Here's how the part is built. I have some questions about the finished solid (model axes, mm). Face numbers are marked on the shaded views. A direction names the side the tool comes from. Coordinates: 2 decimals unless noted, no trailing zeros. Loops run counter-clockwise (first coordinate to the right, second up) from the corner with the lowest first, then second, coordinate; pieces in that order, holes last. Notation, with made-up numbers: M 18.5,-5.75 L 72.5,-5.75 A32 ccw 72.5,29.25 Z; hole C 77.5,-30 d2. An arc over 180 degrees is marked long. Use one line per item in the form item = value. Start each with the question number.
(1) Imagine slicing it at B-B, the plane x = -62. Please give me the cut outline in (y, z).
(2) On a 3-axis mill with a long thin cutter (end or side, diameter ignored), from which of +Z, -Z, +X, -X, +Y, -Y can I reach the whole of each face in a straight line? I mean the marked faces 5 and 6. Say none if no direction works.
(3) Imagine slicing it at D-D, the plane x = -77. Please give me the cut outline in (y, z).
(4) Please list where these lines run through material, in increasing order: L1, parallel to Z at x = -86, y = 3.9; L2, parallel to Z at x = -62, y = 1.55; L3, parallel to X at y = 2.85, z = -12.5.
(5) Imagine slicing it at A-A, the plane z = -12.5. Please give me the cut outline in (x, y), and give its area (3 significant figures).
(6) Imagine slicing it at C-C, the plane y = 3.8. State how many separate pieces and enclosed holes the cut face has, and give its area (3 significant figures).
(7) Thinking about a two-plate mould opening in X: for the marked faces 1, 2, 3 and 4, which applies, +X half, -X half, draft (parallel to the pull), parting line (faces both ways), or undercut?
(8) Will this pin go through, and if not, where does the flat tip stop? P1, Ø3, axis at y = 3, z = -64.5, coming from the +X side.
Autodesk Inventor part; units mm, degrees
ref_plane "YZ Plane" through (0, 0, 0) normal (1, 0, 0) x (0, 1, 0)
ref_plane "XZ Plane" through (0, 0, 0) normal (0, 1, 0) x (-1, 0, 0)
ref_plane "XY Plane" through (0, 0, 0) normal (0, 0, 1) x (1, 0, 0)
sketch "Sketch1" plane through (0, 0, 0) normal (0, 1, 0) x (-1, 0, 0)
  line L0 (0, 0) -> (105, 0)
  line L1 (105, 0) -> (105, -50)
  line L2 (105, -50) -> (0, -50)
  line L3 (0, -50) -> (0, 0)
  line L4 (0, 0) -> (0, -16.6667)
  line L5 (0, -16.6667) -> (11, -16.6667)
  dimension "d0" = 105
  dimension "d1" = 50
  dimension "d2" = 16.6667
  dimension "d3" = 11
extrude "Extrusion1" add sketch "Sketch1" along normal blind 6
sketch "Sketch3" plane through (0, 6, 0) normal (0, 1, 0) x (1, 0, 0)
  circle A0 centre (-20, 12.5) radius 2.75
  line L0 (0, 0) -> (0, 50)
  line L1 (-105, 0) -> (0, 0)
  circle A1 centre (-20, 37.5) radius 2.75
  dimension "d21" = 5.5
  dimension "d22" = 20
  dimension "d23" = 12.5
  dimension "d26" = 25
extrude "Extrusion3" cut sketch "Sketch3" against normal through all
sketch "Sketch4" plane through (0, 6, 0) normal (0, 1, 0) x (1, 0, 0)
  circle A0 centre (-20, 12.5) radius 2.75
  line L0 (-20, 12.5) -> (-78, 12.5)
  line L1 (-78, 12.5) -> (-88, 12.5) construction
  line L2 (-78, 15.25) -> (-88, 15.25)
  line L3 (-88, 9.75) -> (-78, 9.75)
  arc A1 (-78, 9.75) -> (-78, 15.25) centre (-78, 12.5) ccw
  arc A2 (-88, 15.25) -> (-88, 9.75) centre (-88, 12.5) ccw
  point P0 (0, 0)
  point P1 (-83, 12.5)
  dimension "d33" = 58
  dimension "d34" = 10
  dimension "d35" = 5.5
extrude "Extrusion4" cut sketch "Sketch4" against normal through all contours A1 L3 A2 L2
pattern_linear "Rectangular Pattern2" count 2 spacing 25 along (0, 0, -1) of "Extrusion4"
sketch "Sketch5" plane through (0, 0, -50) normal (0, 0, -1) x (-1, 0, 0)
  line L0 (105, 0) -> (105, 6)
  line L1 (105, 0) -> (0, 0)
  line L2 (105, 6) -> (75, 6)
  line L3 (75, 6) -> (75, 0)
  line L4 (75, 0) -> (105, 0)
  line L5 (105, 0) -> (105, 6)
  dimension "d45" = 30
extrude "Extrusion5" add sketch "Sketch5" along normal blind 25
sketch "Sketch6" plane through (0, 6, 0) normal (0, 1, 0) x (1, 0, 0)
  line L0 (-83, 60.5) -> (-83, 70.5) construction
  line L1 (-80.25, 60.5) -> (-80.25, 70.5)
  line L2 (-85.75, 70.5) -> (-85.75, 60.5)
  arc A0 (-85.75, 60.5) -> (-80.25, 60.5) centre (-83, 60.5) ccw
  arc A1 (-80.25, 70.5) -> (-85.75, 70.5) centre (-83, 70.5) ccw
  line L3 (-75, 50) -> (-75, 75)
  arc A2 (-88, 40.25) -> (-88, 34.75) centre (-88, 37.5) ccw
  point P0 (0, 0)
  point P1 (-83, 65.5)
  dimension "d48" = 10
  dimension "d49" = 5.5
  dimension "d50" = 8
  dimension "d51" = 28
extrude "Extrusion6" cut sketch "Sketch6" against normal through all
fillet "Fillet2" radius 5 6 edges at (-105, 3, 0) (0, 3, 0) (-75, 3, -75) (-105, 3, -75) (0, 3, -50) (-75, 3, -50)
sketch "Sketch7" plane through (0, 6, 0) normal (0, 1, 0) x (1, 0, 0)
  circle A0 centre (-20, 12.5) radius 2.75
  line L0 (-20, 12.5) -> (-42, 12.5)
  line L1 (-42, 12.5) -> (-62, 12.5)
  circle A1 centre (-62, 12.5) radius 2.75
  circle A2 centre (-42, 12.5) radius 2.75
  line L2 (0, 5) -> (0, 45)
  line L3 (0, 0) -> (0, 45)
  circle A3 centre (-42, 37.5) radius 2.75
  circle A4 centre (-62, 37.5) radius 2.75
  dimension "d55" = 22
  dimension "d56" = 20
  dimension "d57" = 5.5
  dimension "d58" = 5.5
  dimension "d61" = 25
extrude "Extrusion7" cut sketch "Sketch7" against normal through all contours A2 L1 L0 | L0 L1 A2 | A1 | A3 | A4
sketch "Sketch9" plane through (0, 6, 0) normal (0, 1, 0) x (1, 0, 0)
  point P0 (0, 0)
sketch "Sketch10" plane through (0, 6, 0) normal (0, 1, 0) x (1, 0, 0)
  circle A0 centre (-100, 70) radius 2.75
  line L0 (-100, 75) -> (-80, 75)
  line L1 (-105, 5) -> (-105, 70)
  circle A1 centre (-100, 5) radius 2.75
  line L2 (-100, 0) -> (-5, 0)
  circle A2 centre (-5, 45) radius 2.75
  line L3 (-5, 50) -> (-70, 50)
  line L4 (0, 5) -> (0, 45)
  circle A3 centre (-5, 5) radius 2.75
  point P0 (0, 0)
  dimension "d70" = 5.5
  dimension "d71" = 5
  dimension "d72" = 5
  dimension "d73" = 5.5
  dimension "d74" = 5
  dimension "d75" = 5
  dimension "d76" = 5.5
  dimension "d77" = 5
  dimension "d78" = 5
  dimension "d79" = 5.5
  dimension "d80" = 5
  dimension "d81" = 5
extrude "Extrusion9" cut sketch "Sketch10" against normal through all
sketch "Sketch12" plane through (0, 6, 0) normal (0, 1, 0) x (1, 0, 0)
  circle A0 centre (-42, 37.5) radius 2.75
  line L0 (-42, 37.5) -> (-32, 37.5)
  line L1 (-32, 37.5) -> (-32, 50)
  line L2 (-5, 50) -> (-70, 50)
  line L3 (-32, 50) -> (0, 50)
  line L4 (0, 50) -> (0, 0)
  line L5 (0, 0) -> (-32, 0)
  line L6 (-32, 0) -> (-32, 50)
  dimension "d87" = 10
extrude "Extrusion10" cut sketch "Sketch12" against normal blind 10 contours L1 L2 L3 L4 L5 L6
fillet "Fillet3" radius 5 2 edges at (-32, 3, 0) (-32, 3, -50)
properties part number "X_Carriage_Plate_Short"
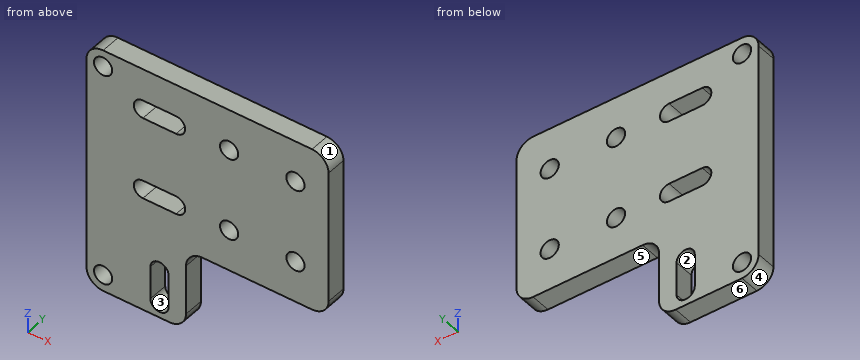
Answer:
q1.outline = M 0,-50 L 6,-50 L 6,-40.25 L 0,-40.25 Z; M 0,-34.75 L 6,-34.75 L 6,-15.25 L 0,-15.25 Z; M 0,-9.75 L 6,-9.75 L 6,0 L 0,0 Z
q2.face_5 = -Z, +X, +Y, -Y
q2.face_6 = -Z, +X, -X, +Y, -Y
q3.outline = M 0,-74 L 6,-74 L 6,-40.06 L 0,-40.06 Z; M 0,-34.94 L 6,-34.94 L 6,-15.06 L 0,-15.06 Z; M 0,-9.94 L 6,-9.94 L 6,0 L 0,0 Z
q4.L1 = -75 to -40.25, -34.75 to -15.25, -9.75 to 0
q4.L2 = -50 to -40.25, -34.75 to -15.25, -9.75 to 0
q4.L3 = -105 to -90.75, -75.25 to -64.75, -59.25 to -44.75, -39.25 to -32
q5.outline = M -105,0 L -90.75,0 L -90.75,6 L -105,6 Z; M -75.25,0 L -64.75,0 L -64.75,6 L -75.25,6 Z; M -59.25,0 L -44.75,0 L -44.75,6 L -59.25,6 Z; M -39.25,0 L -32,0 L -32,6 L -39.25,6 Z
q5.area = 279 mm²
q6.separate_pieces = 1
q6.enclosed_holes = 9
q6.area = 4,000 mm²
q7.face_1 = +X half
q7.face_2 = undercut
q7.face_3 = undercut
q7.face_4 = -X half
q8.P1 = -75
